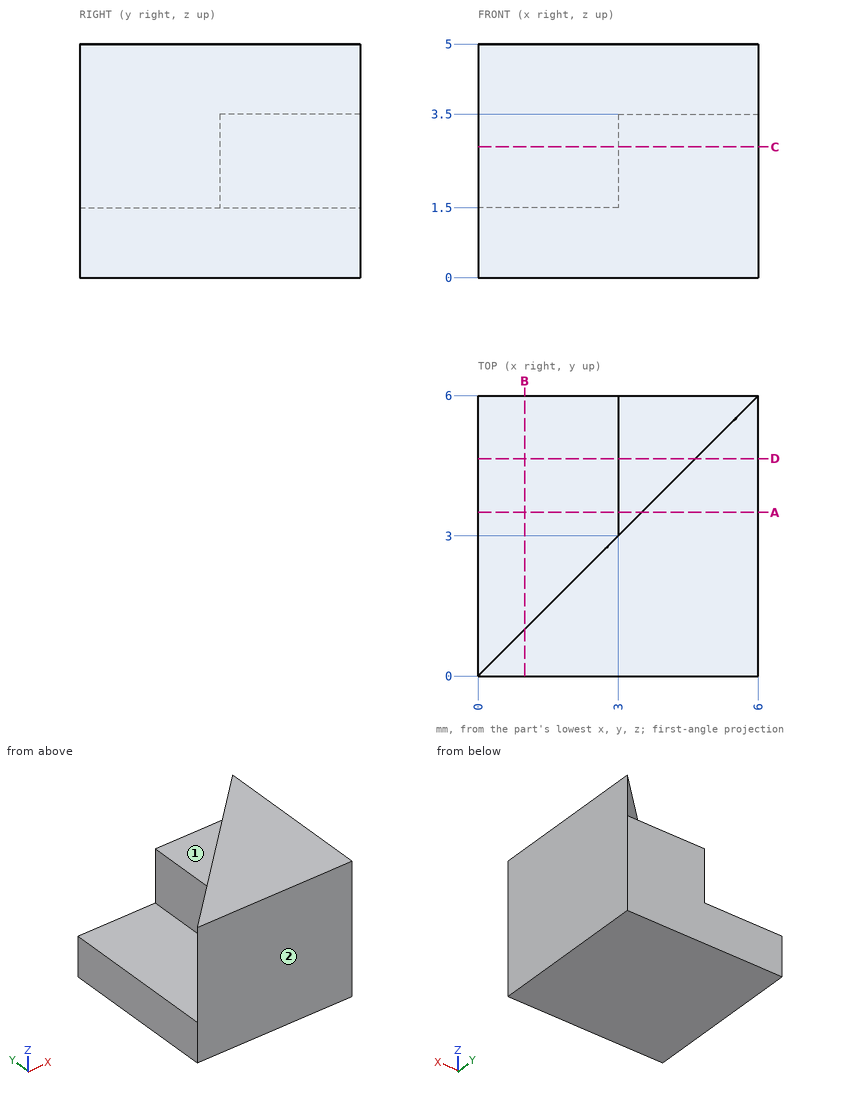
Here's the drawing with two shaded views (mm, measured from the low corner). I have some questions. A direction names the side the tool comes from. Give positions to 0.01 mm unless a question says otherwise; leave off trailing zeros. Loops run counter-clockwise (first coordinate to the right, second up) from the corner with the lowest first, then second, coordinate; pieces in that order, holes last. Notation, with made-up numbers: (66.5, 57.25) - (71.5, 57.25) arc R28 cw to (71.5, 91.25) - close; hole circle Ø7 at (9.25, 79). An arc over 180 degrees is marked (long way). One line per item, written item: value.
(1) I'm going to push flat-ended pins straight in: pin 1 (1 mm diameter, centred on y = 4.5, z = 3, fed in from -X); pin 2 (1 mm diameter, centred on x = 1, y = 4.5, fed in from +Z); pin 3 (1 mm diameter, centred on x = 4, y = 5.5, fed in from +Z). Where does each tip first touch, or does it pass through?
Verdict:
pin 1: x = 3
pin 2: z = 1.5
pin 3: z = 3.5
(2) If we section it at C-C, the plane z = 2.8: List the corners of the cut face in (x, y) for me, plus the area to 3 significant figures.
Verdict:
outline: (0, 0) - (6, 0) - (6, 6) - (3, 6) - (3, 3) - close
area: 22.5 mm^2
(3) On a 3-axis mill with a long thin cutter (end or side, diameter ignored), from which of +Z, -Z, +X, -X, +Y, -Y can I reach the whole of each face in a straight line? I mean the marked faces 1 and 2. Say none if no direction works.
Verdict:
face 1: +Z, -X, +Y
face 2: +Z, -Z, +X, -X, -Y
(4) If we section it at B-B, the plane x = 1: List the corners of the cut face in (y, z) for me, plus the area to 3 significant figures.
Verdict:
outline: (0, 0) - (6, 0) - (6, 1.5) - (1, 1.5) - (1, 5) - (0, 5) - close
area: 12.5 mm^2
(5) If we section it at D-D, the plane y = 4.65: List the corners of the cut face in (x, z) for me, plus the area to 3 significant figures.
Verdict:
outline: (0, 0) - (6, 0) - (6, 5) - (4.65, 5) - (4.65, 3.5) - (3, 3.5) - (3, 1.5) - (0, 1.5) - close
area: 17.0 mm^2
(6) I need wall thicknesses on line 1 along X through (y, z) = (4.4, 2.6); line 2 along Z through (x, y) = (2.3, 5.2); line 3 along X through (y, z) = (2.4, 1.75). Which ranges of each line are inside material? Lowest first, please.
Verdict:
line 1: 3 to 6
line 2: 0 to 1.5
line 3: 2.4 to 6
(7) If we section it at A-A, the plane y = 3.5: List the corners of the cut face in (x, z) for me.
Verdict:
outline: (0, 0) - (6, 0) - (6, 5) - (3.5, 5) - (3.5, 3.5) - (3, 3.5) - (3, 1.5) - (0, 1.5) - close
